For this review, use the dimensioned drawing (mm, ordinates from the lowest corner) and the shaded views. A direction names the side the tool comes from. Coordinates: 2 decimals unless noted, no trailing zeros. Order: outer loops, then holes, each group sorted by start corner. A loop starts at its lowest first (then second) coordinate and runs counter-clockwise, first axis right, second up. Notation, with made-up numbers: (-3, 41.25) -> (24, 41.25) arc R29 cw to (24, 66.25) -> close; hole circle Ø7 at (46.25, -26). An arc over 180 degrees is marked (long way). Return JSON: item names as keys, results as strings. Group by question number.
Item 1: Insertion check: pin 1 (15 mm diameter, centred on x = 19.05, y = 19.05, fed in from +Z); pin 2 (5 mm diameter, centred on x = 5.5, z = 34, fed in from -Y); pin 3 (4 mm diameter, centred on y = 30.5, z = 20.5, fed in from +X). Each pin has a flat end and moves straight along its axis. Give the tip position at first contact, or say it passes through.
Item 2: Take a section at A-A (z = 29). Write out the cut boundary in (x, y) (3 decimals).
Item 3: Machinability: for the marked faces 4, 5, 6 and 7, which of the approach directions +Z, -Z, +X, -X, +Y, -Y give a long, thin tool a straight path to every point of the face, cutting with its end or side? Answer none if there is none.
Item 4: For line 1 along Z through (x, y) = (32, 19); line 2 along Y through (x, z) = (19.05, 14.5) (3 decimals); line 3 along X through (y, z) = (19, 14), list the stretches that pass through material, from the lowest coordinate up.
Item 5: Draft analysis for pull direction Y (two halves, no side actions). For the marked faces 1, 2 and 3, state which applies: +Y half, -Y half, draft (parallel to the pull), parting line (faces both ways), or undercut.
Item 6: Take a section at B-B (x = 17.5). Write out the cut boundary in (y, z), then the cut area to 3 significant figures.
Item 7: Take a section at D-D (y = 21). Write out the cut boundary in (x, z), then the cut area to 3 significant figures.
Item 8: Take a section at C-C (z = 39.5). Write out the cut boundary in (x, y).
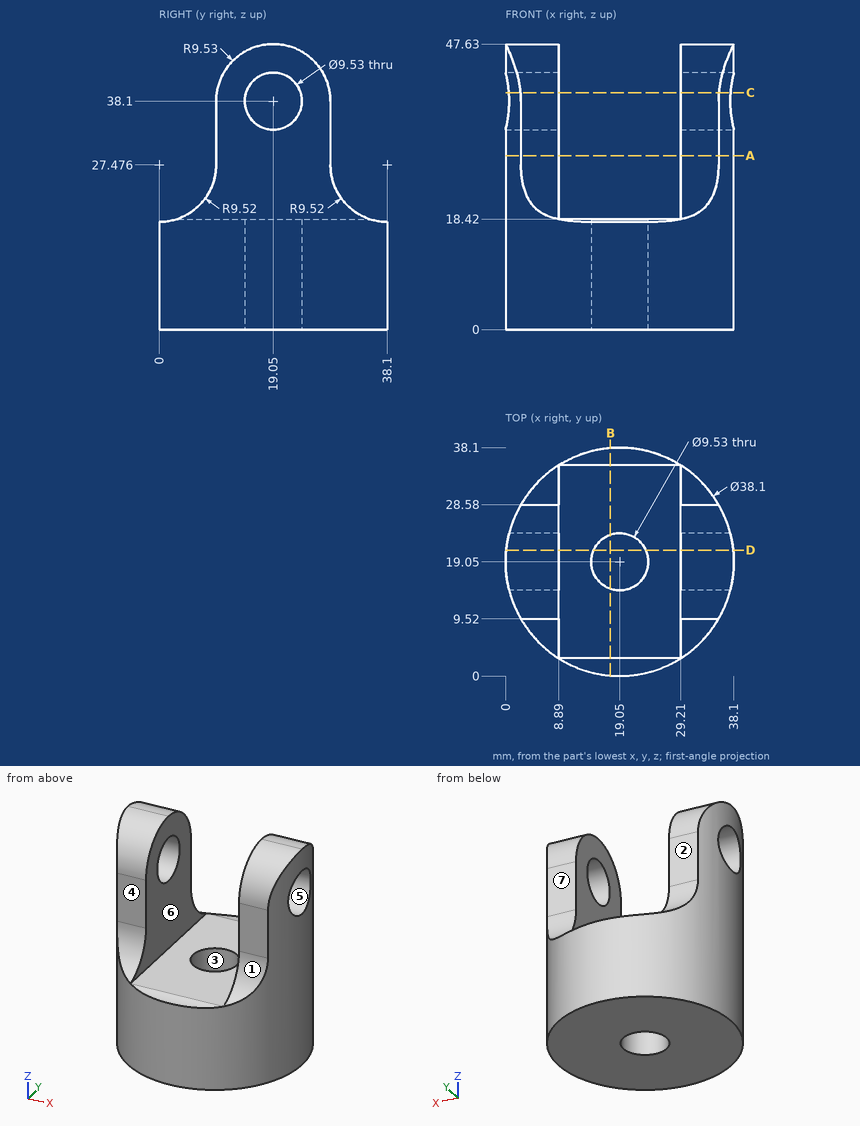
Findings below:
{
 "1": {"pin 1": "stops at z = 18.42", "pin 2": "stops at y = 9.52", "pin 3": "stops at x = 35.59"},
 "2": {"outline": "(2.555, 9.52) -> (8.89, 9.52) -> (8.89, 28.58) -> (2.555, 28.58) arc R19.05 ccw to start; (29.21, 9.52) -> (35.545, 9.52) arc R19.05 ccw to (35.545, 28.58) -> (29.21, 28.58) -> close"},
 "3": {"face 4": "+Z, +X, -X, -Y", "face 5": "+X, -X", "face 6": "+Z, +Y, -Y", "face 7": "+Z, +X, -X, +Y"},
 "4": {"line 1": "z = 0 to 33.34, 42.86 to 47.63", "line 2": "y = 0 to 14.285, 23.815 to 38.1", "line 3": "x = 0 to 14.29, 23.81 to 38.1"},
 "5": {"face 1": "-Y half", "face 2": "+Y half", "face 3": "undercut"},
 "6": {"outline": "(0.06, 0) -> (14.54, 0) -> (14.54, 18.42) -> (2.94, 18.42) arc R9.52 cw to (0.06, 17.96) -> close; (23.56, 0) -> (38.04, 0) -> (38.04, 17.96) arc R9.52 cw to (35.16, 18.42) -> (23.56, 18.42) -> close", "area": "532 mm2"},
 "7": {"outline": "(0.1, 0) -> (14.7, 0) -> (14.7, 18.42) -> (8.89, 18.42) -> (8.89, 33.75) -> (0.1, 33.75) -> close; (0.1, 42.45) -> (8.89, 42.45) -> (8.89, 47.43) -> (0.1, 47.43) -> close; (23.4, 0) -> (38, 0) -> (38, 33.75) -> (29.21, 33.75) -> (29.21, 18.42) -> (23.4, 18.42) -> close; (29.21, 42.45) -> (38, 42.45) -> (38, 47.43) -> (29.21, 47.43) -> close", "area": "895 mm2"},
 "8": {"outline": "(0.55, 14.5) arc R19.05 ccw to (2.5, 9.62) -> (8.89, 9.62) -> (8.89, 14.5) -> close; (0.55, 23.6) -> (8.89, 23.6) -> (8.89, 28.48) -> (2.5, 28.48) arc R19.05 ccw to start; (29.21, 9.62) -> (35.6, 9.62) arc R19.05 ccw to (37.55, 14.5) -> (29.21, 14.5) -> close; (29.21, 23.6) -> (37.55, 23.6) arc R19.05 ccw to (35.6, 28.48) -> (29.21, 28.48) -> close"}
}
